Verification items for this drawing (mm, ordinates from the low corner). A direction names the side the tool comes from. Round coordinates to 2 decimals unless told otherwise and drop trailing zeros. Order: outer loops, then holes, each group sorted by start corner. A loop starts at its lowest first (then second) coordinate and runs counter-clockwise, first axis right, second up.
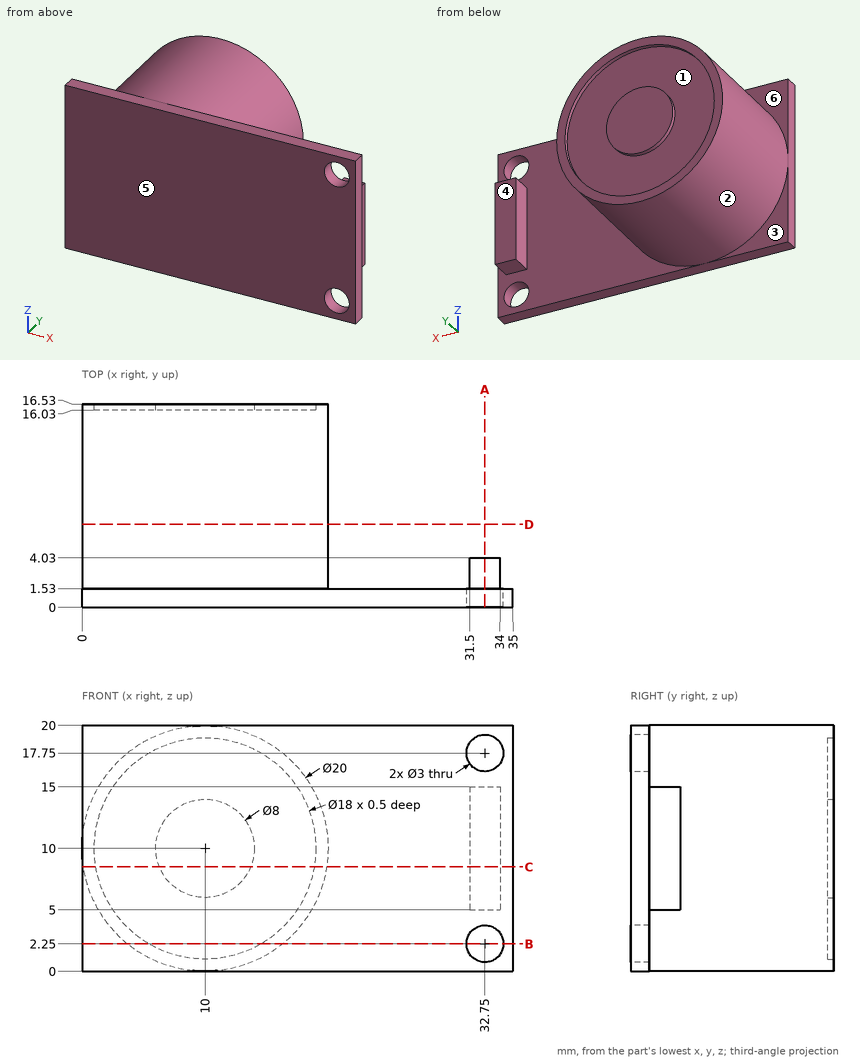
Item 1: Access from +Z, -Z, +X, -X, +Y, -Y to the whole of each face (thin tool, end or side, straight path). Record for the marked faces 4, 5 and 6.
Answer:
face 4: +Z, -Z, +X, +Y
face 5: +Z, -Z, +X, -X, -Y
face 6: +Z, -X, +Y
Item 2: Sectioned sample at C-C (z = 8.5). Record the cut outline in (x, y), and give its area (3 significant figures).
Answer:
outline: (0, 0) - (35, 0) - (35, 1.53) - (34, 1.53) - (34, 4.03) - (31.5, 4.03) - (31.5, 1.53) - (19.89, 1.53) - (19.89, 16.53) - (18.87, 16.53) - (18.87, 16.03) - (13.71, 16.03) - (13.71, 16.53) - (6.29, 16.53) - (6.29, 16.03) - (1.13, 16.03) - (1.13, 16.53) - (0.11, 16.53) - (0.11, 1.53) - (0, 1.53) - close
area: 351 mm2
Item 3: Release check for a two-part mould opening along Z. For the marked faces 1, 2 and 3 record: released by +Z, released by -Z, zero draft, split by the parting line, or undercut.
Answer:
face 1: undercut
face 2: split by the parting line
face 3: zero draft
Item 4: Sectioned sample at D-D (y = 6.75). Record the cut outline in (x, z).
Answer:
outline: circle Ø20 at (10, 10)
Item 5: Sectioned sample at A-A (x = 32.75). Record the cut outline in (y, z).
Answer:
outline: (0, 0) - (1.53, 0) - (1.53, 0.75) - (0, 0.75) - close; (0, 3.75) - (1.53, 3.75) - (1.53, 5) - (4.03, 5) - (4.03, 15) - (1.53, 15) - (1.53, 16.25) - (0, 16.25) - close; (0, 19.25) - (1.53, 19.25) - (1.53, 20) - (0, 20) - close
Item 6: Go/stop test with flat-tipped pins: P1, Ø0.8, axis at x = 33, z = 11, coming from the +Y side; P2, Ø2, axis at x = 33, y = 3.5, coming from the -Z side; P3, Ø4, axis at x = 20.5, z = 18, coming from the +Y side; P4, Ø1.8, axis at x = 32.75, z = 17.75, coming from the +Y side. Record where each tip stops, or that it passes through.
Answer:
P1: stops at y = 4.03
P2: stops at z = 5
P3: stops at y = 1.53
P4: passes through
Item 7: Sectioned sample at B-B (z = 2.25). Record the cut outline in (x, y).
Answer:
outline: (0, 0) - (31.25, 0) - (31.25, 1.53) - (16.32, 1.53) - (16.32, 16.53) - (14.58, 16.53) - (14.58, 16.03) - (5.42, 16.03) - (5.42, 16.53) - (3.68, 16.53) - (3.68, 1.53) - (0, 1.53) - close; (34.25, 0) - (35, 0) - (35, 1.53) - (34.25, 1.53) - close
Item 8: Scan lines: line 1 along Z through (x, y) = (32.75, 0.55); line 2 along X through (y, z) = (16.3, 10). Record each from-to range of solid material in increasing order.
Answer:
line 1: z = 0 to 0.75, 3.75 to 16.25, 19.25 to 20
line 2: x = 0 to 1, 6 to 14, 19 to 20
